from build123d import *

# Parameters (mm, degrees)
SKETCH_1_R      = 4.1
SKETCH_1_R_2    = 1.6
EXTRUDE_1_DEPTH = 7.5


with BuildPart() as part:
    # 草图1 → 凸台-拉伸1 (new body)
    with BuildSketch(Plane.XY):
        Polygon((0, 11.5), (0, 4.5), (0.416202301, 4.5), (28, 4.5), (28, 0), (47, 0), (47, 4.5), (75, 4.5), (75, 18.5), (47, 18.5), (47, 23.5), (28, 23.5), (28, 18.5), (0, 18.5), align=None)
        with Locations((37.5, 11.5)):
            Circle(SKETCH_1_R, mode=Mode.SUBTRACT)
        with Locations((67.5, 11.5)):
            Circle(SKETCH_1_R_2, mode=Mode.SUBTRACT)
        with Locations((32.500024738, 3.227756818)):
            Circle(SKETCH_1_R_2, mode=Mode.SUBTRACT)
        with Locations((42.5, 3.25)):
            Circle(SKETCH_1_R_2, mode=Mode.SUBTRACT)
        with Locations((42.5, 19.75)):
            Circle(SKETCH_1_R_2, mode=Mode.SUBTRACT)
        with Locations((32.500024738, 19.75)):
            Circle(SKETCH_1_R_2, mode=Mode.SUBTRACT)
        with Locations((7.5, 11.5)):
            Circle(SKETCH_1_R_2, mode=Mode.SUBTRACT)
        with Locations((52.370486737, 11.554033831)):
            Circle(SKETCH_1_R_2, mode=Mode.SUBTRACT)
        with Locations((22.5, 11.5)):
            Circle(SKETCH_1_R_2, mode=Mode.SUBTRACT)
    extrude(amount=EXTRUDE_1_DEPTH)


solid = part.part
Model file for the job. Use its own axes, mm. A direction names the side the tool comes from. Give positions to 0.01 mm unless a question says otherwise; leave off trailing zeros. Loops run counter-clockwise (first coordinate to the right, second up) from the corner with the lowest first, then second, coordinate; pieces in that order, holes last.
1) Saw through at C-C (y = 8.75). Write the cut outline in (x, z).
2) Pull direction X, two halves, no side cores. Call faces 1 (the flat face through (0, 12, 4)), 2 (the flat face through (14, 18.5, 4)), 3 (the cylindrical face through (6.32, 12.58, 3.7)): +X half, -X half, draft (parallel to the pull), parting line (faces both ways), or undercut.
3) Flat gauge pins, fed straight in: pin 1 Ø1 at (y, z) = (19.5, 4.5) entering from +X; pin 2 Ø1 at (x, z) = (23.5, 6) entering from -Y; pin 3 Ø2.5 at (y, z) = (20.5, 5.5) entering from -X; pin 4 Ø2.5 at (x, y) = (22.5, 11.5) entering from -Z. Where does each tip first touch, or does it go through?
4) Saw through at D-D (z = 1.75). Count the separate pieces of the cut face and the enclosed holes in it, plus the area to 3 significant figures.
5) Saw through at B-B (x = 42.5). Write the cut outline in (y, z).
6) Saw through at A-A (x = 7.5). Write the cut outline in (y, z), plus the area to 3 significant figures.
7) Tool access for faces 4 (the flat face through (28, 2, 4)), 5 (the flat face through (61, 18.5, 4)), 6 (the flat face through (28, 21, 4)), 7 (the flat face through (61, 4.5, 4)): list every direction of +Z, -Z, +X, -X, +Y, -Y with a clear straight run to the whole face (end or side of a thin tool).
8) Wall check: line 1 (Y direction, x = 37.5, z = 1.75); line 2 (X direction, y = 12, z = 6.25); line 3 (X direction, y = 12.5, z = 2). Give the ranges that are in metal, low to high.
Answer block:
1. outline: (0, 0) - (34.46, 0) - (34.46, 7.5) - (0, 7.5) - close; (40.54, 0) - (75, 0) - (75, 7.5) - (40.54, 7.5) - close
2. face 1: -X half
2. face 2: draft
2. face 3: undercut
3. pin 1: stops at x = 47
3. pin 2: stops at y = 4.5
3. pin 3: stops at x = 28
3. pin 4: passes through
4. separate pieces: 1
4. enclosed holes: 9
4. area: 1,110 mm2
5. outline: (0, 0) - (1.65, 0) - (1.65, 7.5) - (0, 7.5) - close; (4.85, 0) - (18.15, 0) - (18.15, 7.5) - (4.85, 7.5) - close; (21.35, 0) - (23.5, 0) - (23.5, 7.5) - (21.35, 7.5) - close
6. outline: (4.5, 0) - (9.9, 0) - (9.9, 7.5) - (4.5, 7.5) - close; (13.1, 0) - (18.5, 0) - (18.5, 7.5) - (13.1, 7.5) - close
6. area: 81.0 mm2
7. face 4: +Z, -Z, -X, -Y
7. face 5: +Z, -Z, +X, +Y
7. face 6: +Z, -Z, -X, +Y
7. face 7: +Z, -Z, +X, -Y
8. line 1: y = 0 to 7.4, 15.6 to 23.5
8. line 2: x = 0 to 5.98, 9.02 to 20.98, 24.02 to 33.43, 41.57 to 50.83, 53.91 to 65.98, 69.02 to 75
8. line 3: x = 0 to 6.25, 8.75 to 21.25, 23.75 to 33.52, 41.48 to 51.08, 53.66 to 66.25, 68.75 to 75
